Could you check a few things on this drawing? It's one solid part, dimensions in mm from its lowest x, y, z. A direction names the side the tool comes from. Round coordinates to 2 decimals unless told otherwise and drop trailing zeros. Loops run counter-clockwise (first coordinate to the right, second up) from the corner with the lowest first, then second, coordinate; pieces in that order, holes last. Notation, with made-up numbers: (59, 86.25) -> (108, 86.25) arc R23 ccw to (108, 96.25) -> close; hole circle Ø5 at (20, 30.25). An arc over 180 degrees is marked (long way). Put each result on its own line as item: value. Start each with the question number.
1. I'm going to push flat-ended pins straight in: P1, Ø4, axis at x = 87, z = 43, coming from the +Y side; P2, Ø8, axis at x = 130, y = 18.5, coming from the +Z side; P3, Ø20, axis at y = 44.5, z = 33, coming from the -X side. Where does each tip first touch, or does it pass through?
2. Which directions (+Z, -Z, +X, -X, +Y, -Y) give clear straight access to the entire face, cutting with the end or side of a thin tool? Please do the marked faces 5, 6 and 7.
3. I need wall thicknesses on line 1 (X direction, y = 46.5, z = 6); line 2 (Y direction, x = 36, z = 4.5); line 3 (X direction, y = 88.5, z = 33). Which ranges of each line are inside material? Lowest first, please. Write a range as [from, to].
4. Imagine slicing it at A-A, the plane y = 7. Please give me the cut outline in (x, z), and give its area (3 significant figures).
5. If we mould it in two halves opening along X, with no side actions, what happens to the marked faces 1, 2, 3 and 4? For each: pulls with the +X half, pulls with the -X half, needs draft (parallel to the pull), parting line crosses it, or undercut.
6. Imagine slicing it at C-C, the plane x = 33.02. Please give me the cut outline in (y, z).
7. Imagine slicing it at B-B, the plane z = 56. Please give me the cut outline in (x, y) (1 decimal), and give its area (3 significant figures).
8. Imagine slicing it at D-D, the plane y = 38. Please give me the cut outline in (x, z).
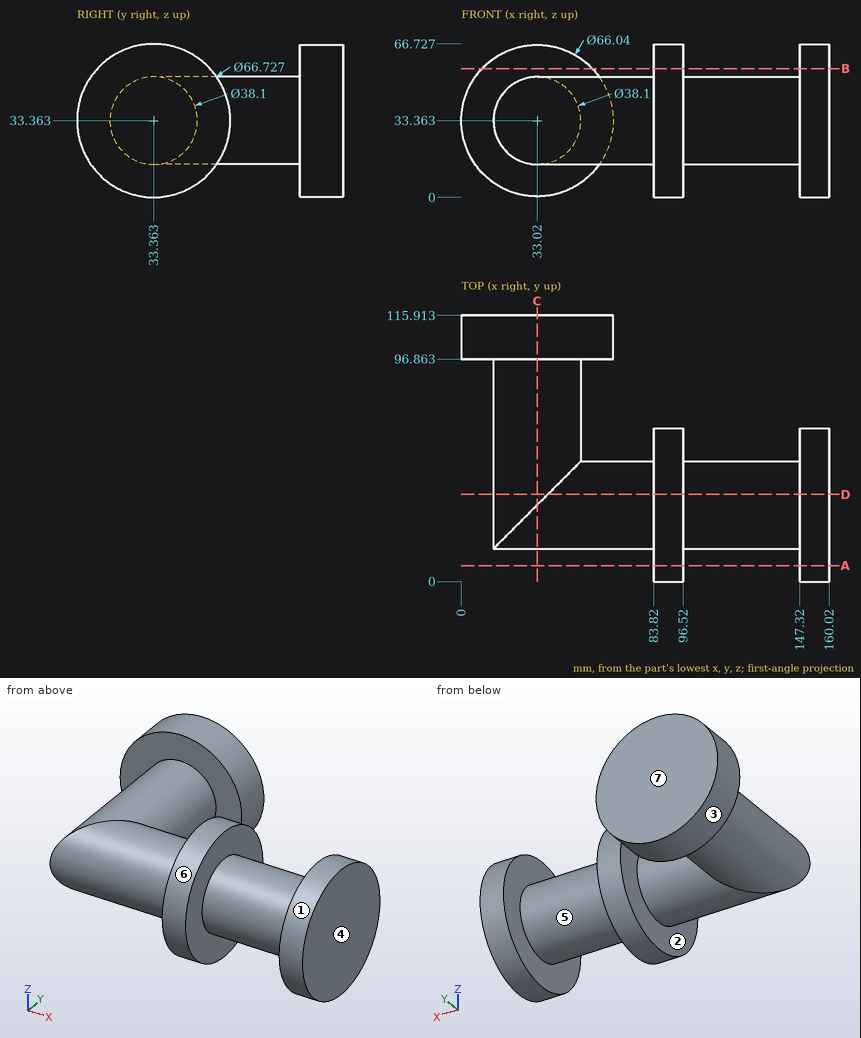
Entries:
1. P1: y = 65.84
1. P2: z = 49.01
1. P3: x = 13.97
2. face 5: none
2. face 6: +X
2. face 7: +Z, -Z, +X, -X, +Y
3. line 1: [83.82, 96.52], [147.32, 160.02]
3. line 2: [96.86, 115.91]
3. line 3: [13.97, 52.07]
4. outline: (83.82, 12.92) -> (96.52, 12.92) -> (96.52, 53.81) -> (83.82, 53.81) -> close; (147.32, 12.92) -> (160.02, 12.92) -> (160.02, 53.81) -> (147.32, 53.81) -> close
4. area: 1,040 mm^2
5. face 1: needs draft
5. face 2: undercut
5. face 3: parting line crosses it
5. face 4: pulls with the +X half
6. outline: (33.36, 14.31) -> (96.86, 14.31) -> (96.86, 0.34) -> (115.91, 0.34) -> (115.91, 66.38) -> (96.86, 66.38) -> (96.86, 52.41) -> (33.36, 52.41) arc R19.05 ccw to start
7. outline: (9, 96.9) -> (57.1, 96.9) -> (57.1, 115.9) -> (9, 115.9) -> close; (83.8, 8.9) -> (96.5, 8.9) -> (96.5, 57.9) -> (83.8, 57.9) -> close; (147.3, 8.9) -> (160, 8.9) -> (160, 57.9) -> (147.3, 57.9) -> close
7. area: 2,160 mm^2
8. outline: (37.66, 14.89) -> (83.82, 14.89) -> (83.82, 0.32) -> (96.52, 0.32) -> (96.52, 14.89) -> (147.32, 14.89) -> (147.32, 0.32) -> (160.02, 0.32) -> (160.02, 66.4) -> (147.32, 66.4) -> (147.32, 51.84) -> (96.52, 51.84) -> (96.52, 66.4) -> (83.82, 66.4) -> (83.82, 51.84) -> (37.66, 51.84) arc R19.05 ccw (long way) to start
